```python
from build123d import *

# Parameters (mm, degrees)
SKETCH_1_R          = 14
EXTRUDE_1_DEPTH     = 4
SKETCH_2_R          = 7.5
EXTRUDE_2_DEPTH     = 14
CUT_EXTRUDE_1_REACH = 28.758
SKETCH_3_R          = 3
CUT_EXTRUDE_2_REACH = 26.249
SKETCH_4_R          = 1.6


with BuildPart() as part:
    # 草图1 → 凸台-拉伸1 (new body)
    with BuildSketch(Plane.XY):
        Circle(SKETCH_1_R)
    extrude(amount=EXTRUDE_1_DEPTH)

    # 草图2 → 凸台-拉伸2 (add)
    with BuildSketch(Plane.XY.offset(4)):
        Circle(SKETCH_2_R)
    extrude(amount=EXTRUDE_2_DEPTH)

    # 草图3 → 切除-拉伸1 (cut, up to next)
    with BuildSketch(Plane.XY.offset(18), mode=Mode.PRIVATE) as cut_extrude_1_sk1:
        Circle(SKETCH_3_R)
    cut_extrude_1_tool1 = extrude(cut_extrude_1_sk1.sketch, amount=-CUT_EXTRUDE_1_REACH, mode=Mode.PRIVATE) & part.part
    add(cut_extrude_1_tool1.solids().sort_by_distance((0, 0, 18))[0], mode=Mode.SUBTRACT)

    # 草图4 → 切除-拉伸2 (cut, up to next)
    with BuildSketch(Plane.XY.offset(4), mode=Mode.PRIVATE) as cut_extrude_2_sk1:
        with Locations((0, 11.5)):
            Circle(SKETCH_4_R)
    cut_extrude_2_tool1 = extrude(cut_extrude_2_sk1.sketch, amount=-CUT_EXTRUDE_2_REACH, mode=Mode.PRIVATE) & part.part
    # 草图4 → 切除-拉伸2 (cut, up to next)
    with BuildSketch(Plane.XY.offset(4), mode=Mode.PRIVATE) as cut_extrude_2_sk2:
        with Locations((9.959292144, 5.75)):
            Circle(SKETCH_4_R)
    cut_extrude_2_tool2 = extrude(cut_extrude_2_sk2.sketch, amount=-CUT_EXTRUDE_2_REACH, mode=Mode.PRIVATE) & part.part
    # 草图4 → 切除-拉伸2 (cut, up to next)
    with BuildSketch(Plane.XY.offset(4), mode=Mode.PRIVATE) as cut_extrude_2_sk3:
        with Locations((9.959292144, -5.75)):
            Circle(SKETCH_4_R)
    cut_extrude_2_tool3 = extrude(cut_extrude_2_sk3.sketch, amount=-CUT_EXTRUDE_2_REACH, mode=Mode.PRIVATE) & part.part
    # 草图4 → 切除-拉伸2 (cut, up to next)
    with BuildSketch(Plane.XY.offset(4), mode=Mode.PRIVATE) as cut_extrude_2_sk4:
        with Locations((0, -11.5)):
            Circle(SKETCH_4_R)
    cut_extrude_2_tool4 = extrude(cut_extrude_2_sk4.sketch, amount=-CUT_EXTRUDE_2_REACH, mode=Mode.PRIVATE) & part.part
    # 草图4 → 切除-拉伸2 (cut, up to next)
    with BuildSketch(Plane.XY.offset(4), mode=Mode.PRIVATE) as cut_extrude_2_sk5:
        with Locations((-9.959292144, -5.75)):
            Circle(SKETCH_4_R)
    cut_extrude_2_tool5 = extrude(cut_extrude_2_sk5.sketch, amount=-CUT_EXTRUDE_2_REACH, mode=Mode.PRIVATE) & part.part
    # 草图4 → 切除-拉伸2 (cut, up to next)
    with BuildSketch(Plane.XY.offset(4), mode=Mode.PRIVATE) as cut_extrude_2_sk6:
        with Locations((-9.959292144, 5.75)):
            Circle(SKETCH_4_R)
    cut_extrude_2_tool6 = extrude(cut_extrude_2_sk6.sketch, amount=-CUT_EXTRUDE_2_REACH, mode=Mode.PRIVATE) & part.part
    add(cut_extrude_2_tool1.solids().sort_by_distance((0, 11.5, 4))[0], mode=Mode.SUBTRACT)
    add(cut_extrude_2_tool2.solids().sort_by_distance((9.959292, 5.75, 4))[0], mode=Mode.SUBTRACT)
    add(cut_extrude_2_tool3.solids().sort_by_distance((9.959292, -5.75, 4))[0], mode=Mode.SUBTRACT)
    add(cut_extrude_2_tool4.solids().sort_by_distance((0, -11.5, 4))[0], mode=Mode.SUBTRACT)
    add(cut_extrude_2_tool5.solids().sort_by_distance((-9.959292, -5.75, 4))[0], mode=Mode.SUBTRACT)
    add(cut_extrude_2_tool6.solids().sort_by_distance((-9.959292, 5.75, 4))[0], mode=Mode.SUBTRACT)


solid = part.part
```
Can you work these out from the model? Positions are in its coordinate system, mm. A direction names the side the tool comes from. Give positions to 0.01 mm unless a question says otherwise; leave off trailing zeros. Loops run counter-clockwise (first coordinate to the right, second up) from the corner with the lowest first, then second, coordinate; pieces in that order, holes last. Notation, with made-up numbers: M 80.5,88.5 L 108.5,88.5 A16 cw 108.5,92.5 Z; hole C -19.5,-4 d9. An arc over 180 degrees is marked long. One line per question, with ' | ' between items. Start each with the question number.
Q1. If we section it at D-D (x = 10): Please give me the cut outline in (y, z), plus the area to 3 significant figures.
Q2. If we section it at A-A (x = 0): Please give me the cut outline in (y, z), plus the area to 3 significant figures.
Q3. If we mould it in two halves opening along Y, with no side actions, what happens to faces 1 (the cylindrical face through (10.7, -7.17, 2.03)), 2 (the flat face through (-0.2, 3.3, 0)), 3 (the cylindrical face through (-7.493, 0.33, 10.902))? For each: +Y half, -Y half, draft (parallel to the pull), parting line (faces both ways), or undercut.
Q4. If we section it at B-B (y = 0): Please give me the cut outline in (x, z), plus the area to 3 significant figures.
Q5. If I drill on line 1 (Y direction, x = 0, z = 1.55); line 2 (Y direction, x = 0, z = 7.75); line 3 (X direction, y = -2.75, z = 15), over which ranges is the centre line in solid material (lowest first)? Write a range as from..to.
Q6. If we section it at C-C (y = -5.75): Please give me the cut outline in (x, z), plus the area to 3 significant figures.
Q7. For pin 1 Ø2.5 at (x, y) = (9.96, 5.75) entering from -Z; pin 2 Ø3.5 at (x, y) = (0, -11.5) entering from +Z; pin 3 Ø2 at (x, z) = (4.5, 13) entering from -Y; pin 4 Ø1 at (x, z) = (0, 6) entering from +Y, each with a flat end and sliding along its axis, tell me the tip position at first contact or that it passes through.
Q8. For faces 4 (the cylindrical face through (-3, 0, 9)), 5 (the flat face through (6, -6, 4)), which set-ups out of +Z, -Z, +X, -X, +Y, -Y let a thin tool reach every point of the face, with its end or its side?
Computed:
1) outline: M -9.8,0 L -7.35,0 L -7.35,4 L -9.8,4 Z; M -4.15,0 L 4.15,0 L 4.15,4 L -4.15,4 Z; M 7.35,0 L 9.8,0 L 9.8,4 L 7.35,4 Z | area: 52.8 mm²
2) outline: M -14,0 L -13.1,0 L -13.1,4 L -14,4 Z; M -9.9,0 L -3,0 L -3,18 L -7.5,18 L -7.5,4 L -9.9,4 Z; M 3,0 L 9.9,0 L 9.9,4 L 7.5,4 L 7.5,18 L 3,18 Z; M 13.1,0 L 14,0 L 14,4 L 13.1,4 Z | area: 188 mm²
3) face 1: undercut | face 2: draft | face 3: parting line
4) outline: M -14,0 L -3,0 L -3,18 L -7.5,18 L -7.5,4 L -14,4 Z; M 3,0 L 14,0 L 14,4 L 7.5,4 L 7.5,18 L 3,18 Z | area: 214 mm²
5) line 1: y = -14..-13.1, -9.9..-3, 3..9.9, 13.1..14 | line 2: y = -7.5..-3, 3..7.5 | line 3: x = -6.98..-1.2, 1.2..6.98
6) outline: M -12.76,0 L -11.56,0 L -11.56,4 L -12.76,4 Z; M -8.36,0 L 8.36,0 L 8.36,4 L 4.82,4 L 4.82,18 L -4.82,18 L -4.82,4 L -8.36,4 Z; M 11.56,0 L 12.76,0 L 12.76,4 L 11.56,4 Z | area: 211 mm²
7) pin 1: passes through | pin 2: stops at z = 4 | pin 3: stops at y = -6.63 | pin 4: stops at y = 7.5
8) face 4: +Z, -Z | face 5: +Z
